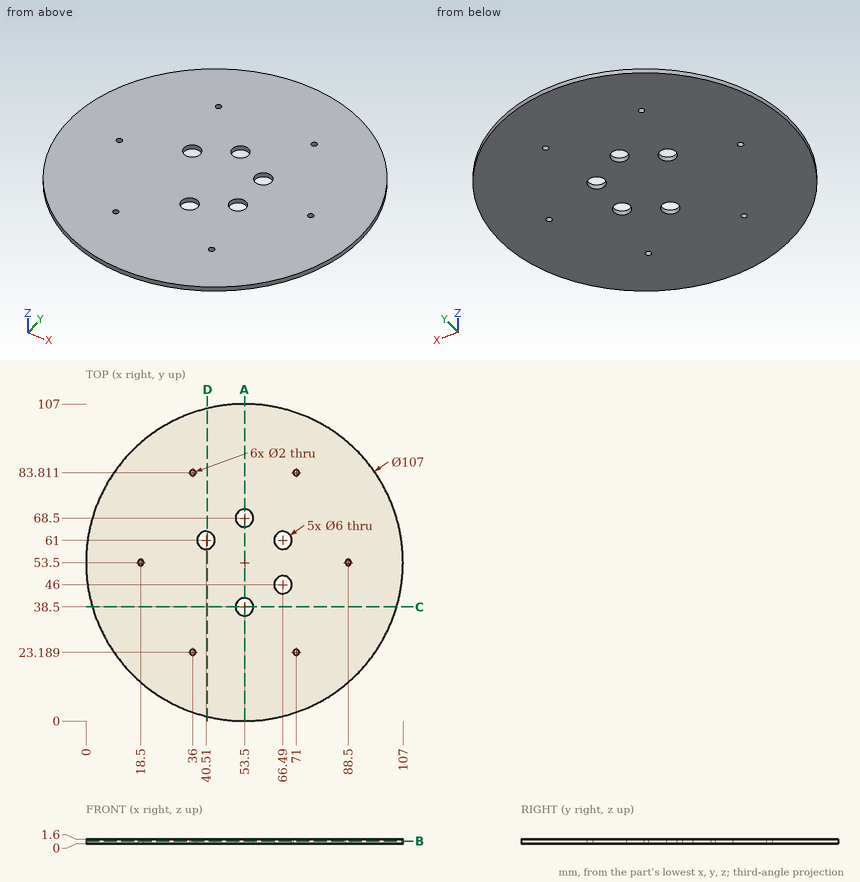
Answer from the drawing. Dimensions are ordinates in mm from the lowest x, y and z of the part. Coordinates: 2 decimals unless noted, no trailing zeros. Write each loop counter-clockwise with the first axis right and the second up, starting at its lowest first coordinate (ties: lowest second). Pieces come first, ordered by that corner, then holes. Notation, with made-up numbers: M 38.25,77 L 78.25,77 A6 ccw 78.25,88 Z; hole C 35.5,-2 d2. An arc over 180 degrees is marked long. Put each result on its own line as item: value. Start each with the question number.
1. A cutting plane is placed at A-A on x = 53.5. Write down the section's boundary in (y, z).
2. A flat-ended cylindrical pin translates along its axis: P1, Ø5.5, axis at x = 66.49, y = 46, coming from the -Z side. Find the tip coordinate at first contact, or state that the pin passes through.
3. A cutting plane is placed at C-C on y = 38.5. Write down the section's boundary in (x, z), then the cut area to 3 significant figures.
4. A cutting plane is placed at B-B on z = 0.9. Count the separate pieces of the cut face and the enclosed holes in it, then the cut area to 3 significant figures.
5. Consider line 1 (Y direction, x = 53.5, z = 0.95); line 2 (Y direction, x = 36, z = 0.55); line 3 (X direction, y = 45.5, z = 0.6). Determine where each line is inside the solid, lowest interval first. Write a range as from..to.
6. A cutting plane is placed at D-D on x = 41. Write down the section's boundary in (y, z).
Resolved:
1. outline: M 0,0 L 35.5,0 L 35.5,1.6 L 0,1.6 Z; M 41.5,0 L 65.5,0 L 65.5,1.6 L 41.5,1.6 Z; M 71.5,0 L 107,0 L 107,1.6 L 71.5,1.6 Z
2. P1: passes through
3. outline: M 2.15,0 L 50.5,0 L 50.5,1.6 L 2.15,1.6 Z; M 56.5,0 L 104.85,0 L 104.85,1.6 L 56.5,1.6 Z
3. area: 155 mm2
4. separate pieces: 1
4. enclosed holes: 11
4. area: 8,830 mm2
5. line 1: y = 0..35.5, 41.5..65.5, 71.5..107
5. line 2: y = 2.94..22.19, 24.19..82.81, 84.81..104.06
5. line 3: x = 0.6..63.53, 69.45..106.4
6. outline: M 1.48,0 L 58.04,0 L 58.04,1.6 L 1.48,1.6 Z; M 63.96,0 L 105.52,0 L 105.52,1.6 L 63.96,1.6 Z
